```python
from build123d import *

# Parameters (mm, degrees)
F0_W     = 393.7
F0_H     = 412.75
F1_DEPTH = 381
F2_W     = 508
F2_H     = 304.8
F3_DEPTH = 3.175
F4_W     = 3.2004
F4_H     = 563.479573
F5_DEPTH = 3.175


with BuildPart() as f1:
    # F0 (on Right) → F1 (new body, symmetric)
    with BuildSketch(Plane.YZ):
        with Locations((-196.85, 206.375)):
            Rectangle(F0_W, F0_H)
    extrude(amount=F1_DEPTH, both=True)

    # F2 (on face) → F3 (cut)
    with BuildSketch(Plane.XZ.offset(393.7)):
        with Locations((-76.2, 209.55)):
            Rectangle(F2_W, F2_H)
    extrude(amount=-F3_DEPTH, mode=Mode.SUBTRACT)

    # F4 (on face) → F5 (cut)
    with BuildSketch(Plane.XZ.offset(393.7)):
        with Locations((230.2002, 202.011388)):
            Rectangle(F4_W, F4_H)
    extrude(amount=-F5_DEPTH, mode=Mode.SUBTRACT)


solid = f1.part
```
Here's how the part is built. I have some questions about the finished solid (model axes, mm). Coordinates: 2 decimals unless noted, no trailing zeros. Return JSON: item names as keys, results as strings.
1) Thinking about a two-plate mould opening in X: for faces 1 (the face through (381, -200, 209)), 2 (the face through (-80, -390.525, 212)), 3 (the face through (-72, -393.7, 20)), which applies, +X half, -X half, draft (parallel to the pull), parting line (faces both ways), or undercut?
Results below:
{"face 1": "+X half", "face 2": "undercut", "face 3": "draft"}
2) I need wall thicknesses on line 1 (Y direction, x = 13, z = 327.5) (3 decimals). Which ranges of the line are inside material? Lowest first, please. Write a range as from..to.
Results below:
{"line 1": "-390.525..0"}
3) Will these pins go through, and if not, where does the flat tip stop? pin 1 (3.5 mm diameter, centred on x = 231, z = 198.5, fed in from -Y); pin 2 (3 mm diameter, centred on x = 3.5, z = 285.5, fed in from -Y) (3 decimals).
Results below:
{"pin 1": "y = -393.7", "pin 2": "y = -390.525"}
